```python
from build123d import *

# Parameters (mm, degrees)
F0_R     = 9
F0_R_2   = 7.5
F1_DEPTH = 8
F2_R     = 9
F3_DEPTH = 1.2
F5_DEPTH = 1


with BuildPart() as f1:
    # F0 (on Top) → F1 (new body)
    with BuildSketch(Plane.XY):
        Circle(F0_R)
        Circle(F0_R_2, mode=Mode.SUBTRACT)
    extrude(amount=F1_DEPTH)

    # F2 (on face) → F3 (join)
    with BuildSketch(Plane.XY.offset(8)):
        Circle(F2_R)
    extrude(amount=F3_DEPTH)

    # F4 (on face) → F5 (join)
    with BuildSketch(Plane.XY.offset(9.2)):
        Polygon((0, 17.7935510874), (-2.3382310135, 8.7057620125), (2.2824784298, 8.7057620125), align=None)
        Polygon((-15.4096672652, 8.8967755437), (-8.7085265689, 2.3279135486), (-6.3981718472, 6.32956531), align=None)
        Polygon((-15.4096672652, -8.8967755437), (-6.3702955553, -6.3778484639), (-8.680650277, -2.3761967025), align=None)
        Polygon((0, -17.7935510874), (2.3382310135, -8.7057620125), (-2.2824784298, -8.7057620125), align=None)
        Polygon((15.4096672652, -8.8967755437), (8.7085265689, -2.3279135486), (6.3981718472, -6.32956531), align=None)
        Polygon((15.4096672652, 8.8967755437), (6.3702955553, 6.3778484639), (8.680650277, 2.3761967025), align=None)
        with BuildLine():
            Line((2.2824784298, 8.7057620125), (-2.2824784298, 8.7057620125))
            ThreePointArc((-2.2824784298, 8.7057620125), (-4.5, 7.7942286341), (-6.3981718472, 6.32956531))
            Line((-6.3981718472, 6.32956531), (-8.680650277, 2.3761967025))
            ThreePointArc((-8.680650277, 2.3761967025), (-9, 0), (-8.680650277, -2.3761967025))
            Line((-8.680650277, -2.3761967025), (-6.3981718472, -6.32956531))
            ThreePointArc((-6.3981718472, -6.32956531), (-4.5, -7.7942286341), (-2.2824784298, -8.7057620125))
            Line((-2.2824784298, -8.7057620125), (2.2824784298, -8.7057620125))
            ThreePointArc((2.2824784298, -8.7057620125), (4.5, -7.7942286341), (6.3981718472, -6.32956531))
            Line((6.3981718472, -6.32956531), (8.680650277, -2.3761967025))
            ThreePointArc((8.680650277, -2.3761967025), (8.9198052807, -1.1987801106), (9, 0))
            ThreePointArc((9, 0), (8.9198052807, 1.1987801106), (8.680650277, 2.3761967025))
            Line((8.680650277, 2.3761967025), (6.3981718472, 6.32956531))
            ThreePointArc((6.3981718472, 6.32956531), (4.5, 7.7942286341), (2.2824784298, 8.7057620125))
        make_face()
    extrude(amount=F5_DEPTH)


solid = f1.part
```
Design review of the part built by this model. Coordinates are the model's own, in mm. A direction names the side the tool comes from. Give positions to 0.01 mm unless a question says otherwise; leave off trailing zeros. Write each loop counter-clockwise with the first axis right and the second up, starting at its lowest first coordinate (ties: lowest second). Pieces come first, ordered by that corner, then holes. Notation, with made-up numbers: (36, 28.5) - (80, 28.5) arc R26 ccw to (80, 57.5) - close; hole circle Ø11 at (42, -31.5). An arc over 180 degrees is marked (long way). Return JSON: item names as keys, results as strings. Group by question number.
(1) We need section B-B, the plane x = 7. Give the boundary of the cut face in (y, z).
(2) We need section A-A, the plane z = 5.75. Give the boundary of the cut face in (x, y), then the cut area to 3 significant figures.
(3) Machinability: for faces 1 (the flat face through (-10.953, -7.655, 9.693)), 2 (the flat face through (-10, 6, 9.2)), 3 (the flat face through (10, -6, 9.2)), 4 (the flat face through (12, 5.59, 9.69)), 5 (the flat face through (-10.841, 7.595, 9.693)), which of the approach directions +Z, -Z, +X, -X, +Y, -Y give a long, thin tool a straight path to every point of the face, cutting with its end or side? Answer none if there is none.
(4) Insertion check: pin 1 (3.5 mm diameter, centred on x = 12.5, y = -4.5, fed in from -Z); pin 2 (4 mm diameter, centred on x = -8, z = 1.5, fed in from -Y); pin 3 (1 mm diameter, centred on x = 7.5, z = 1.5, fed in from -Y). Each pin has a flat end and moves straight along its axis. Give the tip position at first contact, or say it passes through.
(5) Mouldability with a two-part tool opening along Y and no side actions: class faces 6 (the flat face through (-12, -5.59, 9.69)), 7 (the flat face through (-11, -6, 9.2)), 8 (the flat face through (-1.153, 13.313, 9.693)) as +Y half, -Y half, draft (parallel to the pull), parting line (faces both ways), or undercut.
(6) We need section C-C, the plane y = -3.5. Give the boundary of the cut face in (x, z).
(7) We need section D-D, the plane x = -11.5. Give the boundary of the cut face in (y, z).
(8) To check wall thickness, follow probe 1 along Y at (x, z) = (0, 5.75); probe 2 along Z at (x, y) = (-4.5, -2); probe 3 along X at (y, z) = (-1.5, 0.5). State the ranges of each line that lie inside material, in increasing order.
Reported:
{
 "1": {"outline": "(-6.5, 9.2) - (-5.66, 9.2) - (-5.66, 0) - (-2.69, 0) - (-2.69, 8) - (2.69, 8) - (2.69, 0) - (5.66, 0) - (5.66, 9.2) - (6.55, 9.2) - (6.55, 10.2) - (-6.5, 10.2) - close"},
 "2": {"outline": "circle Ø18 at (0, 0); hole circle Ø15 at (0, 0)", "area": "77.8 mm2"},
 "3": {"face 1": "+Z, -Z, -Y", "face 2": "-Z, -X, +Y", "face 3": "-Z, +X, -Y", "face 4": "+Z, -Z, +X", "face 5": "+Z, -Z, +Y"},
 "4": {"pin 1": "stops at z = 9.2", "pin 2": "stops at y = -6.71", "pin 3": "stops at y = -5.66"},
 "5": {"face 6": "undercut", "face 7": "draft", "face 8": "+Y half"},
 "6": {"outline": "(-9.84, 9.2) - (-8.29, 9.2) - (-8.29, 0) - (-6.63, 0) - (-6.63, 8) - (6.63, 8) - (6.63, 0) - (8.29, 0) - (8.29, 9.2) - (9.9, 9.2) - (9.9, 10.2) - (-9.84, 10.2) - close"},
 "7": {"outline": "(-7.81, 9.2) - (-5.11, 9.2) - (-5.11, 10.2) - (-7.81, 10.2) - close; (5.06, 9.2) - (7.78, 9.2) - (7.78, 10.2) - (5.06, 10.2) - close"},
 "8": {"probe 1": "y = -9 to -7.5, 7.5 to 9", "probe 2": "z = 8 to 10.2", "probe 3": "x = -8.87 to -7.35, 7.35 to 8.87"}
}
